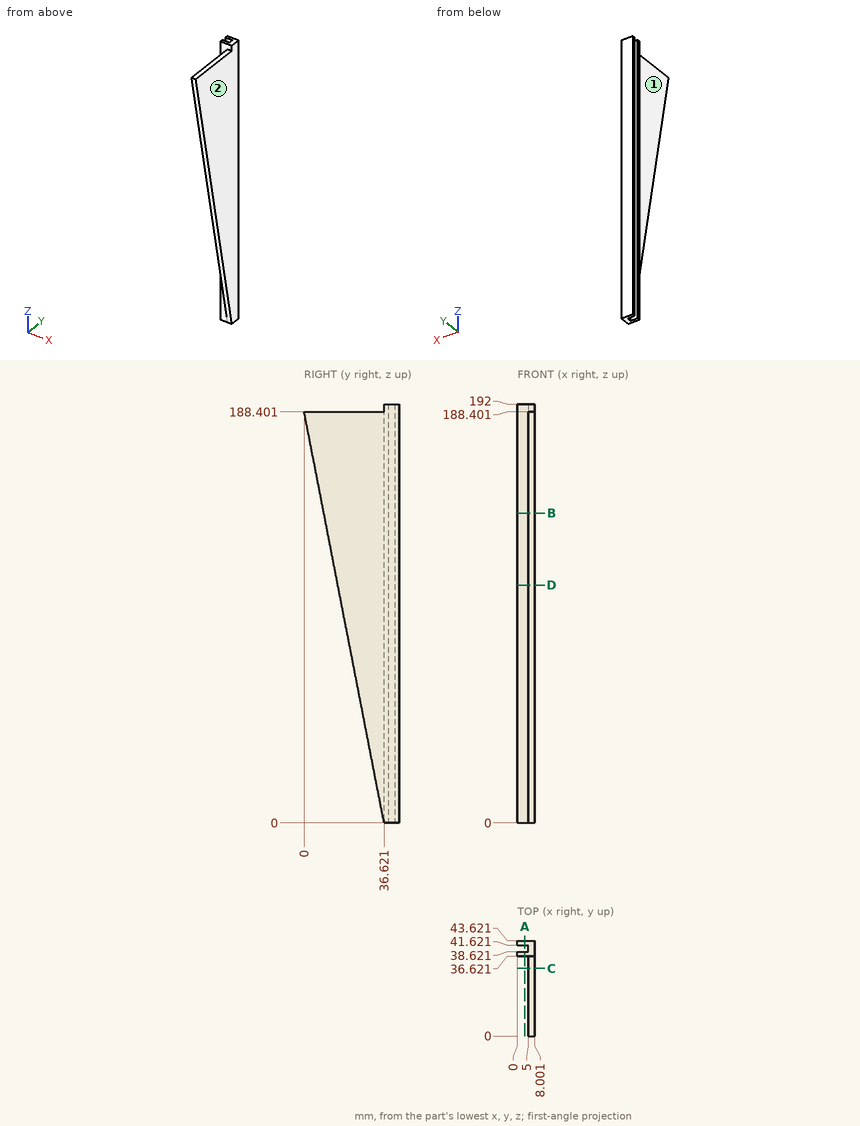
Could you check a few things on this drawing? It's one solid part, dimensions in mm from its lowest x, y, z. A direction names the side the tool comes from. Round coordinates to 2 decimals unless told otherwise and drop trailing zeros. Write each loop counter-clockwise with the first axis right and the second up, starting at its lowest first coordinate (ties: lowest second). Pieces come first, ordered by that corner, then holes. Notation, with made-up numbers: (12, 81.5) -> (55, 81.5) arc R11 ccw to (55, 101.5) -> close; hole circle Ø6 at (4.25, 84). An arc over 180 degrees is marked (long way). Use a Markdown table: item, result.
1. Please list where these lines run through material, in increasing order: probe 1 along Y at (x, z) = (1, 129); probe 2 along X at (y, z) = (36.5, 121); probe 3 along Y at (x, z) = (7.5, 142.5).
Answer key:
| item | result |
|---|---|
| probe 1 | y = 36.62 to 38.62, 41.62 to 43.62 |
| probe 2 | x = 5 to 8 |
| probe 3 | y = 8.92 to 43.62 |
2. If we section it at A-A (x = 3.5): List the corners of the cut face in (y, z) for me.
Answer key:
| item | result |
|---|---|
| outline | (36.62, 0) -> (38.62, 0) -> (38.62, 192) -> (36.62, 192) -> close; (41.62, 0) -> (43.62, 0) -> (43.62, 192) -> (41.62, 192) -> close |
3. If we section it at C-C (y = 31): List the corners of the cut face in (x, z) for me.
Answer key:
| item | result |
|---|---|
| outline | (5, 28.92) -> (8, 28.92) -> (8, 188.4) -> (5, 188.4) -> close |
4. Which directions (+Z, -Z, +X, -X, +Y, -Y) give clear straight access to the entire face, cutting with the end or side of a thin tool? Please do the marked faces 1 and 2.
Answer key:
| item | result |
|---|---|
| face 1 | +Z, -Z, -X, -Y |
| face 2 | +Z, -Z, +X, +Y, -Y |
5. If we section it at D-D (z = 109): List the corners of the cut face in (x, y) for me (1 decimal).
Answer key:
| item | result |
|---|---|
| outline | (0, 36.6) -> (5, 36.6) -> (5, 15.4) -> (8, 15.4) -> (8, 43.6) -> (0, 43.6) -> (0, 41.6) -> (5, 41.6) -> (5, 38.6) -> (0, 38.6) -> close |
6. If we section it at B-B (z = 142): List the corners of the cut face in (x, y) for me, then the cut area to 3 significant figures.
Answer key:
| item | result |
|---|---|
| outline | (0, 36.62) -> (5, 36.62) -> (5, 9.02) -> (8, 9.02) -> (8, 43.62) -> (0, 43.62) -> (0, 41.62) -> (5, 41.62) -> (5, 38.62) -> (0, 38.62) -> close |
| area | 124 mm^2 |
7. For pin 1 Ø11 at (y, z) = (15, 111) entering from -X; pin 2 Ø2.5 at (x, z) = (5.5, 95.5) entering from -Y (1 decimal); pin 3 Ø1.5 at (x, z) = (3, 78.5) entering from -Y; pin 4 Ø2 at (x, y) = (2.5, 22.5) entering from -Z, each with a flat end and sliding along its axis, tell me the tip position at first contact or that it passes through.
Answer key:
| item | result |
|---|---|
| pin 1 | stops at x = 5 |
| pin 2 | stops at y = 17.8 |
| pin 3 | stops at y = 36.62 |
| pin 4 | passes through |
